The figure shows three views and two pictorial views of one solid part (mm, origin at its lowest corner). Answer the questions. Give positions to 0.01 mm unless a question says otherwise; leave off trailing zeros. Order: outer loops, then holes, each group sorted by start corner. A loop starts at its lowest first (then second) coordinate and runs counter-clockwise, first axis right, second up. Notation, with made-up numbers: M -3,39 L 10,39 A28 ccw 10,68 Z; hole C 5,-5 d1. An arc over 180 degrees is marked long. One line per item, written item: value. Start each with the question number.
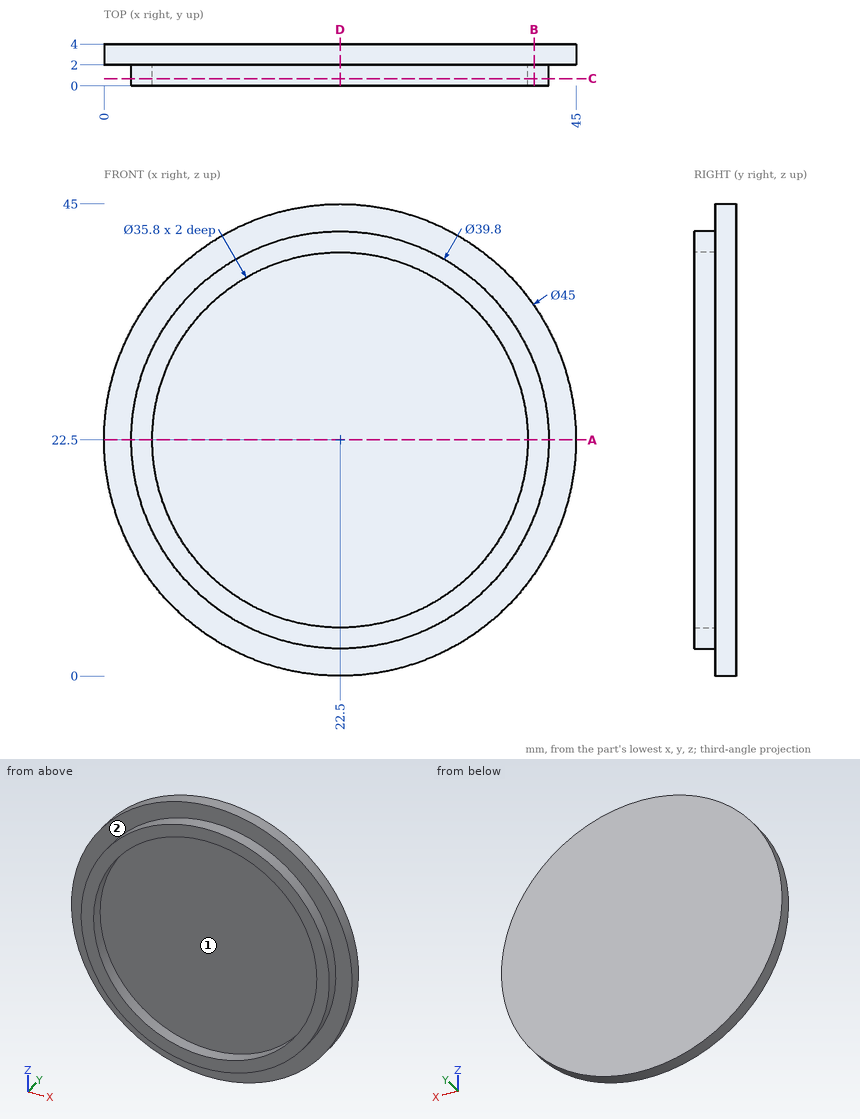
Q1. Consider probe 1 along X at (y, z) = (1.5, 22.5); probe 2 along Y at (x, z) = (30, 2.5); probe 3 along X at (y, z) = (1.05, 26). Determine where each line is inside the solid, lowest interval first.
Q2. Find section C-C, the plane y = 0.7. Give the vertices of the cut face in (x, z), then the cut area to 3 significant figures.
Q3. Find section A-A, the plane z = 22.5. Give the vertices of the cut face in (x, y), then the cut area to 3 significant figures.
Q4. Find section B-B, the plane x = 41. Give the vertices of the cut face in (y, z), then the cut area to 3 significant figures.
Q5. Determine the mould class of the marked faces 1 and 2 for opening direction Z: released by +Z, released by -Z, zero draft, split by the parting line, or undercut.
Q6. Find section D-D, the plane x = 22.5. Give the vertices of the cut face in (y, z).
Q7. Each of these flat-tipped pins is pushed along its axis until it touches: pin 1 (1.5 mm diameter, centred on x = 19, y = 2, fed in from -Z); pin 2 (6 mm diameter, centred on x = 25, z = 17.5, fed in from -Y); pin 3 (4 mm diameter, centred on x = 35, z = 8.5, fed in from -Y); pin 4 (2 mm diameter, centred on y = 2.5, z = 5.5, fed in from +X). Where does it stop, or does it pass through?
Evaluation:
1. probe 1: 2.6 to 4.6, 40.4 to 42.4
1. probe 2: 2 to 4
1. probe 3: 2.91 to 4.95, 40.05 to 42.09
2. outline: C 22.5,22.5 d39.8; hole C 22.5,22.5 d35.8
2. area: 238 mm2
3. outline: M 0,2 L 2.6,2 L 2.6,0 L 4.6,0 L 4.6,2 L 40.4,2 L 40.4,0 L 42.4,0 L 42.4,2 L 45,2 L 45,4 L 0,4 Z
3. area: 98.0 mm2
4. outline: M 0,15.17 L 2,15.17 L 2,9.69 L 4,9.69 L 4,35.31 L 2,35.31 L 2,29.83 L 0,29.83 Z
4. area: 80.6 mm2
5. face 1: undercut
5. face 2: zero draft
6. outline: M 0,2.6 L 2,2.6 L 2,0 L 4,0 L 4,45 L 2,45 L 2,42.4 L 0,42.4 L 0,40.4 L 2,40.4 L 2,4.6 L 0,4.6 Z
7. pin 1: z = 0.17
7. pin 2: y = 2
7. pin 3: y = 0
7. pin 4: x = 38.32
